```python
from build123d import *
from build123d.topology import SkipClean

# Parameters (mm, degrees)
BOSS_EXTRUDE1_DEPTH = 6
BOSS_EXTRUDE2_START = 7
BOSS_EXTRUDE2_DEPTH = 7
SKETCH3_R           = 2.5
CUT_EXTRUDE1_DEPTH  = 7
CUT_EXTRUDE2_REACH  = 84.35
SKETCH5_R           = 51
CUT_EXTRUDE3_DEPTH  = 2


with BuildPart() as part:
    # Sketch1 → Boss-Extrude1 (new body)
    with BuildSketch(Plane(origin=(0, 0, 0), x_dir=(0, 0, -1), z_dir=(1, 0, 0))):
        with BuildLine():
            Line((-57, 7.566372975), (-57, -7.566372975))
            ThreePointArc((-57, -7.566372975), (57.5, 0), (-57, 7.566372975))
        make_face()
    extrude(amount=BOSS_EXTRUDE1_DEPTH)

    # Sketch2 → Boss-Extrude2 (add)
    with SkipClean():  # the faces are left unmerged after this step: merging them gives an invalid solid
        with BuildSketch(Plane.ZY.offset(BOSS_EXTRUDE2_START)):
            with BuildLine():
                Line((-29.380225594, -41.686956522), (-33.12476415, -47))
                ThreePointArc((-33.12476415, -47), (23.049066289, -52.678179004), (57, -7.566372975))
                Line((57, -7.566372975), (57, 7.566372975))
                ThreePointArc((57, 7.566372975), (23.049066289, 52.678179004), (-33.12476415, 47))
                Line((-33.12476415, 47), (-29.380225594, 41.686956522))
                ThreePointArc((-29.380225594, 41.686956522), (20.443519665, 46.723254421), (50.556521739, 6.711043856))
                ThreePointArc((50.556521739, 6.711043856), (50.889009662, 3.362840414), (51, 0))
                ThreePointArc((51, 0), (50.889009662, -3.362840414), (50.556521739, -6.711043856))
                ThreePointArc((50.556521739, -6.711043856), (20.443519665, -46.723254421), (-29.380225594, -41.686956522))
            make_face()
        extrude(amount=-BOSS_EXTRUDE2_DEPTH)

    # Sketch3 → Cut-Extrude1 (cut)
    with SkipClean():  # the faces are left unmerged after this step: merging them gives an invalid solid
        with BuildSketch(Plane.XY.offset(57)):
            with Locations((-2, 0)):
                Circle(SKETCH3_R)
        extrude(amount=-CUT_EXTRUDE1_DEPTH, mode=Mode.SUBTRACT)

    # Sketch4 → Cut-Extrude2 (cut, up to next)
    with BuildSketch(Plane(origin=(6, 0, 0), x_dir=(0, 0, -1), z_dir=(1, 0, 0)), mode=Mode.PRIVATE) as cut_extrude2_sk1:
        with BuildLine():
            ThreePointArc((-44.60706125, -5.933808779), (44.999999572, 0.006203806), (-44.608695652, 5.921509285))
            ThreePointArc((-44.608695652, 5.921509285), (-45, 0), (-44.608695652, -5.921509285))
            ThreePointArc((-44.608695652, -5.921509285), (-44.607878875, -5.927659088), (-44.60706125, -5.933808779))
        make_face()
    cut_extrude2_tool1 = extrude(cut_extrude2_sk1.sketch, amount=-CUT_EXTRUDE2_REACH, mode=Mode.PRIVATE) & part.part
    add(cut_extrude2_tool1.solids().sort_by_distance((6, 0, 0))[0], mode=Mode.SUBTRACT)

    # Sketch5 → Cut-Extrude3 (cut)
    with SkipClean():  # the faces are left unmerged after this step: merging them gives an invalid solid
        with BuildSketch(Plane.ZY):
            with Locations(Location((0, 0, 0), (0, 0, 234.824499503))):
                Circle(SKETCH5_R)
        extrude(amount=-CUT_EXTRUDE3_DEPTH, mode=Mode.SUBTRACT)


solid = part.part
```
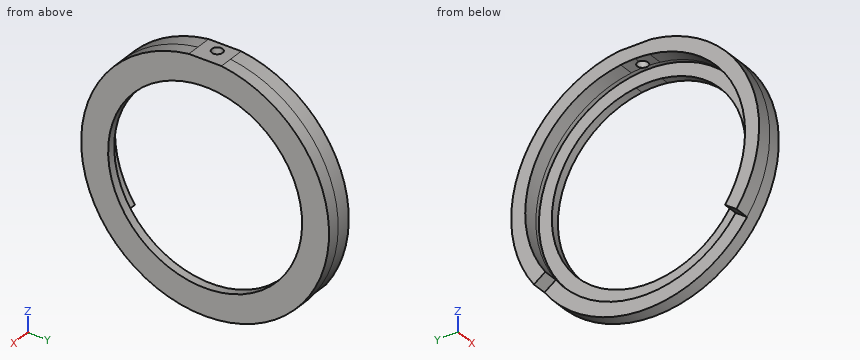
Design review of the part built by this model. Coordinates are the model's own, in mm. Coordinates: 2 decimals unless noted, no trailing zeros. Loops run counter-clockwise (first coordinate to the right, second up) from the corner with the lowest first, then second, coordinate; pieces in that order, holes last. Notation, with made-up numbers: M 63.25,13.5 L 93.25,13.5 A27 ccw 93.25,35.5 Z; hole C 9.5,-37 d7. An arc over 180 degrees is marked long. One line per question, with ' | ' between items.
(1) We need section B-B (z = 0). Give the boundary of the cut face in (x, y), and give its area (3 significant figures).
Filled in:
outline: M -7,-57.5 L 6,-57.5 L 6,-45 L 2,-45 L 2,-51 L -7,-51 Z; M -7,51 L 2,51 L 2,45 L 6,45 L 6,57.5 L -7,57.5 Z | area: 217 mm^2
(2) We need section A-A (x = -2). Give the boundary of the cut face in (y, z).
Filled in:
outline: M -47,-33.12 L -41.69,-29.38 A51 cw -2.5,50.94 L -2.5,57 L -7.57,57 A57.5 ccw Z; M 2.5,50.94 A51 cw 41.69,-29.38 L 47,-33.12 A57.5 ccw 7.57,57 L 2.5,57 Z
(3) We need section C-C (y = 28). Give the boundary of the cut face in (x, z).
Filled in:
outline: M -7,42.63 L 2,42.63 L 2,35.23 L 6,35.23 L 6,50.22 L -7,50.22 Z; M 0,-50.22 L 6,-50.22 L 6,-35.23 L 2,-35.23 L 2,-42.63 L 0,-42.63 Z
(4) Wall thickness on probe 1 along Y at (x, z) = (4.45, 0); probe 2 along X at (y, z) = (0, 54); probe 3 along Y at (x, z) = (0.9, 0): over which ranges is each line inside the solid? List them lowest first.
Filled in:
probe 1: y = -57.5 to -45, 45 to 57.5 | probe 2: x = -7 to -4.5, 0.5 to 6 | probe 3: y = -57.5 to -51, 51 to 57.5
(5) For pin 1 Ø4 at (x, z) = (-1.5, 32.5) entering from -Y; pin 2 Ø5 at (x, z) = (4.5, -25.5) entering from -Y; pin 3 Ø5 at (x, z) = (0.5, 19) entering from +Y, all flat-tipped, find the tip position at first contact; note any pin that passes through.
Filled in:
pin 1: stops at y = -48.74 | pin 2: stops at y = -52.7 | pin 3: stops at y = 55.08
